Design review of the part built by this model. Coordinates are the model's own, in mm. Give positions to 0.01 mm unless a question says otherwise; leave off trailing zeros. Order: outer loops, then holes, each group sorted by start corner. A loop starts at its lowest first (then second) coordinate and runs counter-clockwise, first axis right, second up. Notation, with made-up numbers: (-34.5, 70) -> (-8.5, 70) arc R23 ccw to (-8.5, 93) -> close; hole circle Ø4 at (47.25, 69.5). An arc over 180 degrees is marked (long way). One line per item, written item: value. Start each with the question number.
1) Consider section D-D (x = 55). State the section outline as (y, z) points (3 decimals), plus the area to 3 significant figures.
2) For pin 1 (11.5 mm diameter, centred on x = -101.6, y = 0, fed in from +Z) (3 decimals); pin 2 (1.5 mm diameter, centred on y = -32, z = 2.5, fed in from +X), all flat-tipped, find the tip position at first contact; note any pin that passes through.
3) Consider section A-A (z = 2.6). State the section outline as (x, y) points, plus the area to 3 significant figures.
4) The part is to be moulded in two halves that separate along Y. For faces 1 (the face through (-31, 1, 0)), 2 (the face through (-71.865, -45.171, 1.565)), 3 (the face through (-111.243, 0.424, 1.565)), 4 (the face through (-70.682, 45.704, 1.565)), say which applies: released by +Y, released by -Y, zero draft, split by the parting line, or undercut.
5) Wall thickness on line 1 along X through (y, z) = (2.5, 0.9); line 2 along X through (y, z) = (5.5, 0.25); line 3 along Y through (x, z) = (-101.6, 1.15): over which ranges is each line inside the solid? List them lowest first. Write a range as from..to.
6) Consider section C-C (y = -56). State the section outline as (x, z) points (3 decimals), plus the area to 3 significant figures.
7) Consider section B-B (x = -101.6). State the section outline as (y, z) points (3 decimals), plus the area to 3 significant figures.
from build123d import *

# Parameters (mm, degrees)
F0_R     = 13.9065
F0_R_2   = 9.652
F1_DEPTH = 3.175


# Not quite as in the source:
# - a length typed as a fraction of an inch, garbled in the dataset ("3 / 203.2 mm" for 3/8 in), is restored


with BuildPart() as f1:
    # F0 (on Top) → F1 (new body)
    with BuildSketch(Plane.XY):
        with BuildLine():
            Line((-29.0468705796, 64.4645603781), (-113.5004093806, 26.4109228888))
            ThreePointArc((-113.5004093806, 26.4109228888), (-130.5681996552, 0), (-113.5004093806, -26.4109228888))
            Line((-113.5004093806, -26.4109228888), (-29.0468705796, -64.4645603781))
            ThreePointArc((-29.0468705796, -64.4645603781), (70.706437014, 0), (-29.0468705796, 64.4645603781))
        make_face()
        with Locations((-101.6, 0)):
            Circle(F0_R, mode=Mode.SUBTRACT)
        with BuildLine():
            ThreePointArc((0, 64.77), (45.7993062175, 45.7993062175), (64.77, 0))
            ThreePointArc((64.77, 0), (45.7993062175, -45.7993062175), (0, -64.77))
            ThreePointArc((0, -64.77), (-45.7993062175, -45.7993062175), (-64.77, 0))
            ThreePointArc((-64.77, 0), (-45.7993062175, 45.7993062175), (0, 64.77))
        make_face(mode=Mode.SUBTRACT)
        with Locations((-101.6, 0)):
            Circle(F0_R)
        with Locations((-101.6, 0)):
            Circle(F0_R_2, mode=Mode.SUBTRACT)
        with BuildLine():
            Line((0, 9.652), (0, 64.77))
            ThreePointArc((0, 64.77), (-45.7993062175, 45.7993062175), (-64.77, 0))
            Line((-64.77, 0), (-9.652, 0))
            ThreePointArc((-9.652, 0), (-6.824994652, 6.824994652), (0, 9.652))
        make_face()
        with BuildLine():
            ThreePointArc((-64.77, 0), (-45.7993062175, -45.7993062175), (0, -64.77))
            Line((0, -64.77), (0, -9.652))
            ThreePointArc((0, -9.652), (-6.824994652, -6.824994652), (-9.652, 0))
            Line((-9.652, 0), (-64.77, 0))
        make_face()
        with BuildLine():
            ThreePointArc((0, -64.77), (45.7993062175, -45.7993062175), (64.77, 0))
            ThreePointArc((64.77, 0), (45.7993062175, 45.7993062175), (0, 64.77))
            Line((0, 64.77), (0, 9.652))
            ThreePointArc((0, 9.652), (6.824994652, 6.824994652), (9.652, 0))
            ThreePointArc((9.652, 0), (6.824994652, -6.824994652), (0, -9.652))
            Line((0, -9.652), (0, -64.77))
        make_face()
    extrude(amount=F1_DEPTH)


solid = f1.part
Checked values:
1. outline: (-44.434, 0) -> (44.434, 0) -> (44.434, 3.175) -> (-44.434, 3.175) -> close
1. area: 282 mm^2
2. pin 1: passes through
2. pin 2: stops at x = 63.43
3. outline: (-113.5, -26.41) -> (-29.05, -64.46) arc R70.71 ccw (long way) to (-29.05, 64.46) -> (-113.5, 26.41) arc R28.97 ccw to start; hole circle Ø19.3 at (-101.6, 0); hole circle Ø19.3 at (0, 0)
3. area: 19,600 mm^2
4. face 1: zero draft
4. face 2: released by -Y
4. face 3: undercut
4. face 4: released by +Y
5. line 1: x = -130.46..-110.92, -92.28..-9.32, 9.32..70.66
5. line 2: x = -130.04..-109.53, -93.67..-7.93, 7.93..70.49
5. line 3: y = -31.77..-9.65, 9.65..31.77
6. outline: (-47.833, 0) -> (43.167, 0) -> (43.167, 3.175) -> (-47.833, 3.175) -> close
6. area: 289 mm^2
7. outline: (-31.773, 0) -> (-9.652, 0) -> (-9.652, 3.175) -> (-31.773, 3.175) -> close; (9.652, 0) -> (31.773, 0) -> (31.773, 3.175) -> (9.652, 3.175) -> close
7. area: 140 mm^2
